Model file for the job. Use its own axes, mm. A direction names the side the tool comes from. Give positions to 0.01 mm unless a question says otherwise; leave off trailing zeros. Write each loop counter-clockwise with the first axis right and the second up, starting at its lowest first coordinate (ties: lowest second). Pieces come first, ordered by that corner, then holes.
Autodesk Fusion 360 part; units mm, degrees
sketch "Sketch1" plane through (0, 0, 0) normal (0, 1, 0) x (1, 0, 0)
  line L0 (20, -20) -> (-20, -20)
  line L1 (-20, -20) -> (-20, 20)
  line L2 (-20, 20) -> (20, 20)
  line L3 (20, 20) -> (20, -20)
  line L4 (20, -20) -> (-20, 20) construction
  line L5 (-20, -20) -> (20, 20) construction
  line L6 (-20, 4) -> (-15, 4)
  line L7 (-15, 4) -> (-15, -4)
  line L8 (-15, -4) -> (-20, -4)
  line L9 (-20, -4) -> (-20, 4)
  line L10 (-4, 20) -> (4, 20)
  line L11 (4, 20) -> (4, 15)
  line L12 (4, 15) -> (-4, 15)
  line L13 (-4, 15) -> (-4, 20)
  line L14 (20, 4) -> (15, 4)
  line L15 (15, 4) -> (15, -4)
  line L16 (15, -4) -> (20, -4)
  line L17 (20, -4) -> (20, 4)
  line L18 (-4, -20) -> (4, -20)
  line L19 (4, -20) -> (4, -15)
  line L20 (4, -15) -> (-4, -15)
  line L21 (-4, -15) -> (-4, -20)
  dimension "d1" = 40
  dimension "d2" = 40
  dimension "d3" = 5
  dimension "d4" = 8
  dimension "d5" = 16
  dimension "d6" = 5
  dimension "d7" = 16
  dimension "d8" = 8
  dimension "d9" = 5
  dimension "d10" = 5
  dimension "d11" = 8
  dimension "d12" = 8
  dimension "d13" = 16
  dimension "d14" = 16
extrude "Extrude1" add sketch "Sketch1" against normal blind 3 contours L0 L1 L2 L3 L6 L7 L8 L11 L12 L13 L14 L15 L16 L19 L20 L21
extrude "Extrude2" add sketch "Sketch1" against normal blind 8 contours L0 L18 L19 L20 L21 | L3 L14 L15 L16 L17 | L1 L6 L7 L8 L9 | L2 L10 L11 L12 L13
hole "Hole1" at (0, 0, 0) direction (0, -1, 0) diameter 9 depth 30 tip angle 118
fillet "Fillet1" radius 4 4 edges at (20, -1.5, -20) (-20, -1.5, -20) (20, -1.5, 20) (-20, -1.5, 20)
sketch "Sketch2" plane through (0, 0, 0) normal (0, 0, 1) x (1, 0, 0)
sketch "Sketch3" plane through (0, 0, 0) normal (0, 1, 0) x (1, 0, 0)
  line L0 (-10.5, 20) -> (10.5, 20)
  line L1 (10.5, 20) -> (10.5, 8)
  line L2 (10.5, 8) -> (-10.5, 8)
  line L3 (-10.5, 8) -> (-10.5, 20)
  line L4 (-20, -20) -> (-20, 20)
  dimension "d26" = 21
  dimension "d27" = 9.5
  dimension "d28" = 12
extrude "Extrude3" add sketch "Sketch3" along normal blind 80
sketch "Sketch4" plane through (0, 0, -8) normal (0, 0, 1) x (1, 0, 0)
  line L0 (-10.5, 0) -> (10.5, 0)
  line L1 (10.5, 0) -> (10.5, 80)
  line L2 (10.5, 80) -> (-10.5, 80)
  line L3 (-10.5, 80) -> (-10.5, 0)
  line L4 (-10.5, 80) -> (10.5, 80)
  line L5 (10.5, 80) -> (10.5, 59)
  line L6 (10.5, 59) -> (-10.5, 59)
  line L7 (-10.5, 59) -> (-10.5, 80)
  line L8 (8.5, 78) -> (8.5, 61)
  line L9 (8.5, 61) -> (-8.5, 61)
  line L10 (-8.5, 61) -> (-8.5, 78)
  line L11 (-8.5, 78) -> (8.5, 78)
  line L12 (-8.5, 78) -> (8.5, 78)
  line L13 (8.5, 78) -> (8.5, 64.8708)
  line L14 (-8.5, 64.8708) -> (-8.5, 78)
  line L15 (-8.5, 61) -> (8.5, 61)
  line L16 (8.5, 61) -> (8.5, 70.3993)
  line L17 (8.5, 70.3993) -> (-8.5, 70.3993)
  line L18 (-8.5, 70.3993) -> (-8.5, 61)
  point P0 (-7.5, 64)
  point P1 (7.5, 64)
  dimension "d29" = 21
  dimension "d30" = 21
  dimension "d31" = 2
  dimension "d34" = 5
  dimension "d35" = 15
  dimension "d36" = 3
extrude "Extrude5" cut sketch "Sketch4" against normal blind 3 contours L8 L9 L10 L13 L14 L15 L16 L17 L18
sketch "Sketch6" plane through (0, 0, -20) normal (0, 0, -1) x (-1, 0, 0)
  line L0 (16, -3) -> (16, 0)
  line L1 (16, 0) -> (10.5, 0)
  line L2 (10.5, 0) -> (10.5, 80)
  line L3 (10.5, 80) -> (-10.5, 80)
  line L4 (-10.5, 80) -> (-10.5, 0)
  line L5 (-10.5, 0) -> (-16, 0)
  line L6 (-16, 0) -> (-16, -3)
  line L7 (-16, -3) -> (-4, -3)
  line L8 (-4, -3) -> (-4, -8)
  line L9 (-4, -8) -> (4, -8)
  line L10 (4, -8) -> (4, -3)
  line L11 (4, -3) -> (16, -3)
  point P0 (-7.5, 75)
  point P1 (7.5, 75)
  dimension "d45" = 15
  dimension "d46" = 3
  dimension "d47" = 5
hole "Hole4" at (7.5, 75, -20) at (-7.5, 75, -20) direction (0, 0, 1) diameter 3 depth 12 tip angle 118 counterbore diameter 5 counterbore depth 9
equation "d6 = d3"
equation "d7 = d5"
equation "d8 = d4"
equation "d9 = d3"
equation "d10 = d3"
equation "d11 = d4"
equation "d12 = d4"
equation "d13 = d7"
equation "d14 = d7"
1. Slice it at D-D, the plane x = 2. Write the cut outline in (y, z).
Calculated:
outline: (-8, -20) - (80, -20) - (80, -8) - (70.4, -8) - (70.4, -11) - (61, -11) - (61, -8) - (0, -8) - (0, -4.03) - (-3, -4.03) - (-3, -15) - (-8, -15) - close; (-8, 15) - (-3, 15) - (-3, 4.03) - (0, 4.03) - (0, 20) - (-8, 20) - close
2. Pin check, flat tips, straight feed: P1, Ø2.5, axis at y = -6.5, z = 17.5, coming from the +X side; P2, Ø1.5, axis at x = 18.5, y = -4.5, coming from the -Z side; P3, Ø3, axis at x = -13.5, z = 11.5, coming from the +Y side. Stop position of each tip, or through.
Calculated:
P1: stops at x = 4
P2: stops at z = -4
P3: stops at y = 0
3. Pull direction X, two halves, no side cores. Call faces 1 (the flat face through (0, 66, -11)), 2 (the flat face through (20, -3, 0)), 3 (the flat face through (0, -5, 15)), 4 (the flat face through (-20, -3, 0)): +X half, -X half, draft (parallel to the pull), parting line (faces both ways), or undercut.
Calculated:
face 1: undercut
face 2: +X half
face 3: draft
face 4: -X half
4. Probe probe 1 along X at (y, z) = (75, -10.2); probe 2 along Y at (x, z) = (-7.5, -9.3); probe 3 along X at (y, z) = (75, -17.5). List the from-to ranges inside material, lowest first.
Calculated:
probe 1: x = -10.5 to -9, -6 to 6, 9 to 10.5
probe 2: y = -3 to 61, 70.4 to 73.5, 76.5 to 80
probe 3: x = -10.5 to -10, -5 to 5, 10 to 10.5
5. Which spindle directions (+Z, -Z, +X, -X, +Y, -Y) get a long thin tool onto all of the face, cutting with end or side? Do faces 5 (the flat face through (17, -5, 4)), 6 (the flat face through (4, -5, -18)), 7 (the flat face through (-18, -5, -4)), 8 (the flat face through (0, 61, -9)), 9 (the flat face through (15, -5, 0)). Say none if no direction does.
Calculated:
face 5: +Z, +X, -X, -Y
face 6: +Z, -Z, +X, -Y
face 7: -Z, +X, -X, -Y
face 8: +Z
face 9: +Z, -Z, -Y
6. Slice it at A-A, the plane y = 75. Write the cut outline in (x, z), and give its area (3 significant figures).
Calculated:
outline: (-10.5, -20) - (-10, -20) - (-10, -11) - (-9, -11) - (-9, -8) - (-10.5, -8) - close; (-6, -11) - (-5, -11) - (-5, -20) - (5, -20) - (5, -11) - (6, -11) - (6, -8) - (-6, -8) - close; (9, -11) - (10, -11) - (10, -20) - (10.5, -20) - (10.5, -8) - (9, -8) - close
area: 144 mm2
7. Slice it at B-B, the plane x = -7.5. Write the cut outline in (y, z), and give its area (3 significant figures).
Calculated:
outline: (-3, -20) - (72.5, -20) - (72.5, -11) - (73.5, -11) - (73.5, -8) - (70.4, -8) - (70.4, -11) - (61, -11) - (61, -8) - (0, -8) - (0, 20) - (-3, 20) - close; (76.5, -11) - (77.5, -11) - (77.5, -20) - (80, -20) - (80, -8) - (76.5, -8) - close
area: 998 mm2
8. Slice it at C-C, the plane z = 0. Write the cut outline in (x, y).
Calculated:
outline: (-20, -8) - (-15, -8) - (-15, -3) - (-4.5, -3) - (-4.5, 0) - (-20, 0) - close; (4.5, -3) - (15, -3) - (15, -8) - (20, -8) - (20, 0) - (4.5, 0) - close
